Check sheet for the modelled part. Datum: model origin and axes. Units: mm. Face numbers are marked on the shaded views. Give positions to 0.01 mm unless a question says otherwise; leave off trailing zeros. Order: outer loops, then holes, each group sorted by start corner. A loop starts at its lowest first (then second) coordinate and runs counter-clockwise, first axis right, second up. Notation, with made-up numbers: (-29, -34) -> (-11, -34) arc R31 cw to (-11, -6) -> close; hole circle Ø1 at (85, 67.5). An arc over 180 degrees is marked (long way). One line per question, with ' | ' between items.
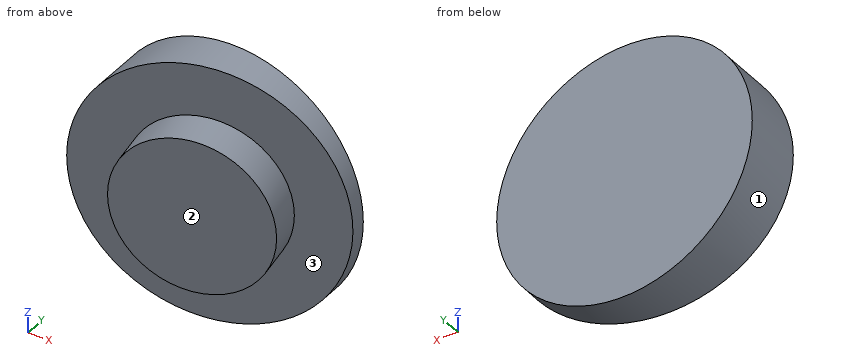
```python
from build123d import *

# Parameters (mm, degrees)
SKETCH_5_R          = 25
EXTRUDE_4_DEPTH     = 20
CUT_EXTRUDE_2_DEPTH = 41
SKETCH_8_R          = 15
EXTRUDE_5_DEPTH     = 7


with BuildPart() as part:
    # 草图5 → 凸台-拉伸4 (new body)
    with BuildSketch(Plane(origin=(0, 0, 0), x_dir=(1, 0, 0), z_dir=(0, 1, 0))):
        Circle(SKETCH_5_R)
    extrude(amount=EXTRUDE_4_DEPTH)

    # 草图7 → 切除-拉伸2 (cut, symmetric)
    with BuildSketch(Plane.XY):
        Polygon((-25, 8.183650965), (25, 17), (25, -9.727272727), (-25, -9.727272727), align=None)
    extrude(amount=CUT_EXTRUDE_2_DEPTH, both=True, mode=Mode.SUBTRACT)

    # 草图8 → 凸台-拉伸5 (add)
    with BuildSketch(Plane(origin=(-2.153328978, 12.212135485, 0), x_dir=(0.984807753, 0.173648178, 0), z_dir=(0.173648178, -0.984807753, 0))):
        with Locations((2.186547548, 0)):
            Circle(SKETCH_8_R)
    extrude(amount=EXTRUDE_5_DEPTH)


solid = part.part
```
Q1. Depth check by flat-ended pin: pin 1 Ø1 at (y, z) = (9.5, 9) entering from +X; pin 2 Ø8 at (x, y) = (17.5, 15.5) entering from +Z; pin 3 Ø1 at (x, y) = (10.5, 18) entering from -Z. Enter the tip coordinate at first touch or a pass-through.
Result sheet:
pin 1: stops at x = 13.11 | pin 2: stops at z = 21.04 | pin 3: stops at z = -22.91
Q2. Mould release check, pull along X, two halves, no side actions. Record for the marked faces 1, 2 and 3: pulls with the +X half, pulls with the -X half, needs draft (parallel to the pull), parting line crosses it, or undercut.
Result sheet:
face 1: parting line crosses it | face 2: pulls with the +X half | face 3: undercut
Q3. Section check A-A (z = 0). Enter the section's corners in (x, y), and give its area (3 significant figures).
Result sheet:
outline: (-25, 8.18) -> (-14.77, 9.99) -> (-13.56, 3.09) -> (15.99, 8.3) -> (14.77, 15.2) -> (25, 17) -> (25, 20) -> (-25, 20) -> close | area: 580 mm2
Q4. Section check C-C (y = 16). Enter the section's corners in (x, z).
Result sheet:
outline: (19.33, -15.86) -> (19.33, 15.86) arc R25 ccw (long way) to start
Q5. Section check B-B (x = -19.5). Enter the section's corners in (y, z), and give its area (3 significant figures).
Result sheet:
outline: (9.15, -15.64) -> (20, -15.64) -> (20, 15.64) -> (9.15, 15.64) -> close | area: 339 mm2
Q6. Section check D-D (z = 14). Enter the section's corners in (x, y), and give its area (3 significant figures).
Result sheet:
outline: (-20.71, 8.94) -> (-5.3, 11.66) -> (-4.09, 4.76) -> (6.52, 6.63) -> (5.3, 13.53) -> (20.71, 16.24) -> (20.71, 20) -> (-20.71, 20) -> close | area: 382 mm2
Q7. Thickness scan on line 1 (Z direction, x = -8, y = 8); line 2 (Z direction, x = 15.5, y = 17); line 3 (Y direction, x = 10, z = 5.5). Record the ranges inside material, lowest first.
Result sheet:
line 1: z = -12.24 to 12.24 | line 2: z = -19.62 to 19.62 | line 3: y = 7.25 to 20
